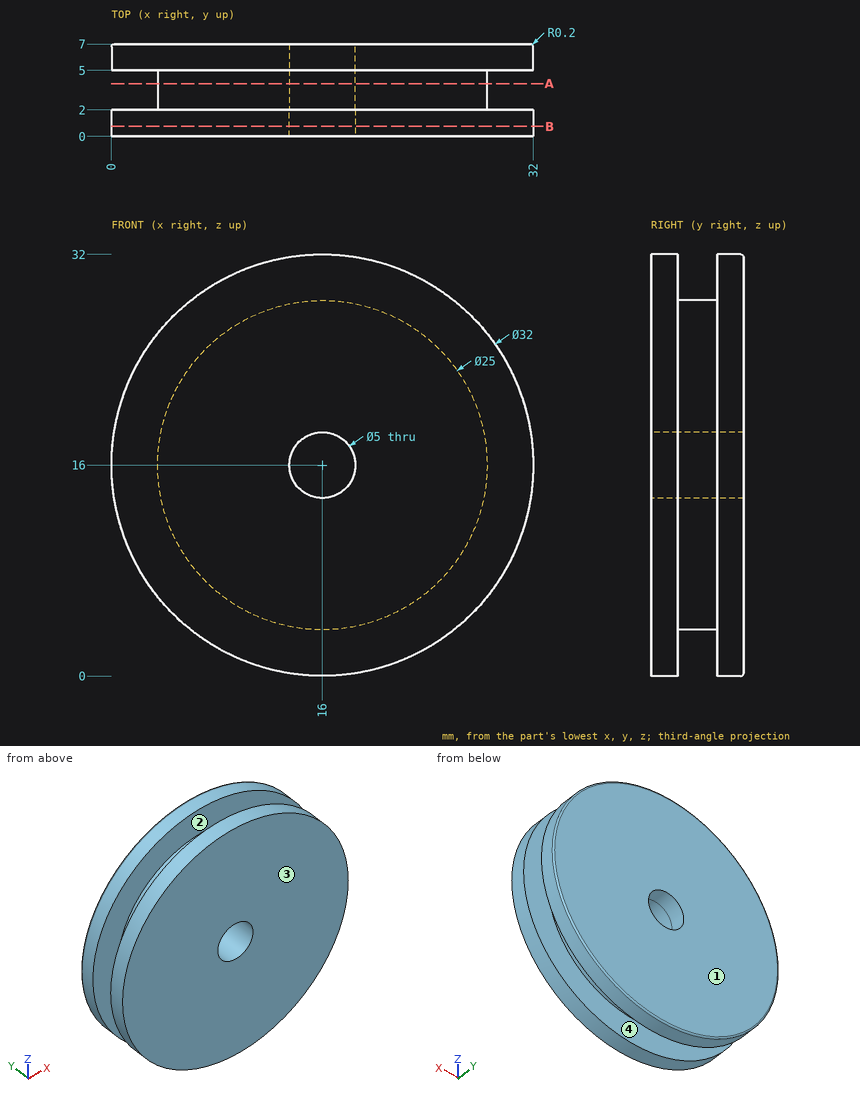
Part print with two shaded views. Sizes in mm from the minimum x, y, z corner. Coordinates: 2 decimals unless noted, no trailing zeros. Write each loop counter-clockwise with the first axis right and the second up, starting at its lowest first coordinate (ties: lowest second). Pieces come first, ordered by that corner, then holes. Notation, with made-up numbers: (44, -20) - (78, -20) arc R24 cw to (78, 13) - close; hole circle Ø1 at (59, 21). An arc over 180 degrees is marked (long way). Use a Markdown table: item, result. Add a question column.
Item 1: Two-plate mould, pull along Y, no slides. Class the marked faces 1, 2, 3 and 4: pulls with the +Y half, pulls with the -Y half, needs draft (parallel to the pull), parting line crosses it, or undercut.
Item 2: Drill centre lines: line 1 along Y through (x, z) = (18.5, 1); line 2 along X through (y, z) = (3.55, 16); line 3 along Z through (x, y) = (16, 6.6). Where is each one in solid material? Low to high.
Item 3: Drop flat-ended pins along their axis: pin 1 (1 mm diameter, centred on y = 5.5, z = 7, fed in from +X); pin 2 (4 mm diameter, centred on x = 17, y = 2.5, fed in from -Z); pin 3 (3 mm diameter, centred on x = 4, y = 5.5, fed in from +Z); pin 4 (3 mm diameter, centred on x = 6, y = 1, fed in from +Z). Give the stop position or say it passes through.
Item 4: Band-saw the part on A-A, the plane y = 4. Write the cut outline in (x, z).
Item 5: Band-saw the part on B-B, the plane y = 0.75. Write the cut outline in (x, z), and give its area (3 significant figures).
A:
| question | item | result |
|---|---|---|
| 1 | face 1 | pulls with the +Y half |
| 1 | face 2 | undercut |
| 1 | face 3 | pulls with the -Y half |
| 1 | face 4 | undercut |
| 2 | line 1 | y = 0 to 2, 5 to 7 |
| 2 | line 2 | x = 3.5 to 13.5, 18.5 to 28.5 |
| 2 | line 3 | z = 0 to 13.5, 18.5 to 32 |
| 3 | pin 1 | stops at x = 29.56 |
| 3 | pin 2 | stops at z = 0 |
| 3 | pin 3 | stops at z = 28.07 |
| 3 | pin 4 | stops at z = 29.56 |
| 4 | outline | circle Ø25 at (16, 16); hole circle Ø5 at (16, 16) |
| 5 | outline | circle Ø32 at (16, 16); hole circle Ø5 at (16, 16) |
| 5 | area | 785 mm² |
